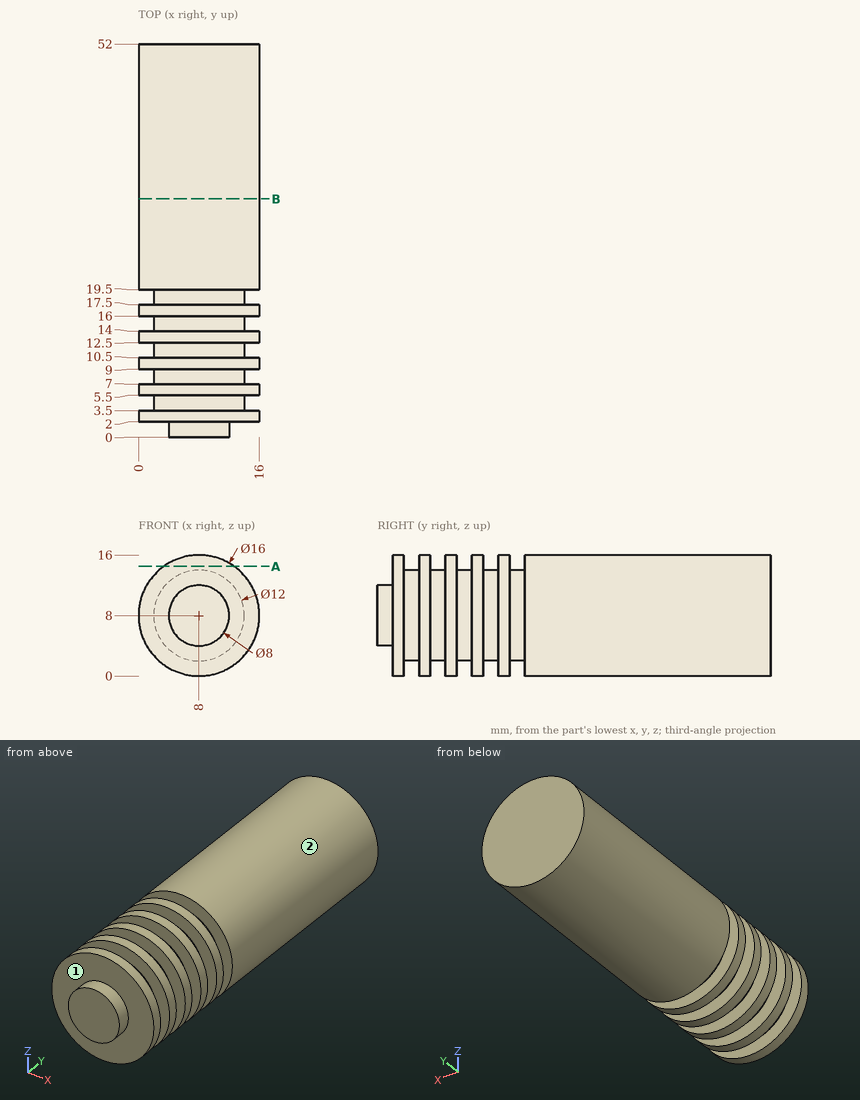
Geometry check sheet. Reference: drawing and pictorial views, mm from the part's lowest x, y, z. A direction names the side the tool comes from. Coordinates: 2 decimals unless noted, no trailing zeros. Order: outer loops, then holes, each group sorted by start corner. A loop starts at its lowest first (then second) coordinate and runs counter-clockwise, first axis right, second up. Notation, with made-up numbers: (41.25, 20) - (96.25, 20) arc R5 cw to (96.25, 29) - close; hole circle Ø3 at (-4.75, -18.5). An arc over 180 degrees is marked (long way). Answer in a Markdown table with one row per item. Add a question column.
1) Cross-section at B-B, the plane y = 31.5. Record the cut outline in (x, z).
2) Set-up check for the marked faces 1 and 2: record each of +Z, -Z, +X, -X, +Y, -Y from which the full face is reachable in a straight line by a thin tool's end or side.
3) Material ranges on line 1 along Y through (x, z) = (3.25, 13.5); line 2 along Y through (x, z) = (3, 9); line 3 along Z through (x, y) = (11.5, 32.5), recorded low to high. Write a range as [from, to].
4) Gauge pin test, flat ends, axial feed: P1, Ø1.5, axis at x = 12.5, y = 12, coming from the +Z side; P2, Ø1, axis at x = 6, z = 14, coming from the -Y side; P3, Ø5, axis at y = 17.5, z = 7, coming from the -X side; P4, Ø1.5, axis at x = 10.5, y = 6, coming from the -Z side. Record the tip position at first contact, or that the pin passes through.
5) Cross-section at A-A, the plane z = 14.5. Record the cut outline in (x, y), then the cut area to 3 significant figures.
Check result:
| question | item | result |
|---|---|---|
| 1 | outline | circle Ø16 at (8, 8) |
| 2 | face 1 | -Y |
| 2 | face 2 | +Y, -Y |
| 3 | line 1 | y = [2, 3.5], [5.5, 7], [9, 10.5], [12.5, 14], [16, 17.5], [19.5, 52] |
| 3 | line 2 | y = [2, 52] |
| 3 | line 3 | z = [0.81, 15.19] |
| 4 | P1 | stops at z = 14.96 |
| 4 | P2 | stops at y = 2 |
| 4 | P3 | stops at x = 0 |
| 4 | P4 | stops at z = 0.19 |
| 5 | outline | (3.34, 2) - (12.66, 2) - (12.66, 3.5) - (3.34, 3.5) - close; (3.34, 5.5) - (12.66, 5.5) - (12.66, 7) - (3.34, 7) - close; (3.34, 9) - (12.66, 9) - (12.66, 10.5) - (3.34, 10.5) - close; (3.34, 12.5) - (12.66, 12.5) - (12.66, 14) - (3.34, 14) - close; (3.34, 16) - (12.66, 16) - (12.66, 17.5) - (3.34, 17.5) - close; (3.34, 19.5) - (12.66, 19.5) - (12.66, 52) - (3.34, 52) - close |
| 5 | area | 373 mm² |
